from build123d import *

# Parameters (mm, degrees)
F1_DEPTH = 2165
F2_W     = 1270
F2_H     = 45
F3_DEPTH = 40
F4_W     = 925
F4_H     = 2125
F5_DEPTH = 235


with BuildPart() as f1:
    # F0 (on Top) → F1 (new body)
    with BuildSketch(Plane.XY):
        Polygon((0, 255), (0, 0), (1270, 0), (1270, 45), (965, 45), (965, 255), align=None)
    extrude(amount=F1_DEPTH)

    # F2 (on face) → F3 (join)
    with BuildSketch(Plane.XY.offset(2165)):
        with Locations((635, 22.5)):
            Rectangle(F2_W, F2_H)
    extrude(amount=F3_DEPTH)

    # F4 (on face) → F5 (cut)
    with BuildSketch(Plane.XZ):
        with Locations((482.5, 1082.5)):
            Rectangle(F4_W, F4_H)
    extrude(amount=-F5_DEPTH, mode=Mode.SUBTRACT)


solid = f1.part
CAD build for the part. Positions are in the model's coordinates, mm. A direction names the side the tool comes from. Coordinates: 2 decimals unless noted, no trailing zeros. Order: outer loops, then holes, each group sorted by start corner. A loop starts at its lowest first (then second) coordinate and runs counter-clockwise, first axis right, second up.
Item 1: Two-plate mould, pull along Z, no slides. Class faces 1 (the face through (485, 129, 0)), 2 (the face through (1055, 0, 1179)), 3 (the face through (476, 116, 20)), 4 (the face through (476, 151, 2165)): +Z half, -Z half, draft (parallel to the pull), parting line (faces both ways), or undercut.
Check sheet entries:
face 1: -Z half
face 2: draft
face 3: undercut
face 4: +Z half
Item 2: Band-saw the part on B-B on x = 268. List the corners of the cut face in (y, z).
Check sheet entries:
outline: (0, 0) - (255, 0) - (255, 2165) - (45, 2165) - (45, 2205) - (0, 2205) - (0, 2145) - (235, 2145) - (235, 20) - (0, 20) - close
Item 3: Drill centre lines: L1, parallel to Z at x = 707, y = 84; L2, parallel to X at y = 226, z = 1235.5; L3, parallel to Z at x = 943.5, y = 22.5. Where is each one in solid material? Low to high.
Check sheet entries:
L1: z = 0 to 20, 2145 to 2165
L2: x = 0 to 20, 945 to 965
L3: z = 0 to 20, 2145 to 2205
Item 4: Pin check, flat tips, straight feed: pin 1 Ø3 at (y, z) = (84.5, 1675) entering from +X; pin 2 Ø4 at (x, y) = (631.5, 93) entering from +Z. Stop position of each tip, or through.
Check sheet entries:
pin 1: stops at x = 965
pin 2: stops at z = 2165
Item 5: 3-axis set-ups, long thin cutter, end or side, ignore diameter. For faces 5 (the face through (945, 116, 1068)), 6 (the face through (965, 149, 1067)), 7 (the face through (626, 23, 2205)): which of +Z, -Z, +X, -X, +Y, -Y reach the whole face in a straight line?
Check sheet entries:
face 5: -Y
face 6: +Z, -Z, +X, +Y
face 7: +Z, +X, -X, +Y, -Y
Item 6: Band-saw the part on A-A on z = 331. List the corners of the cut face in (x, y), plus the area to 3 significant figures.
Check sheet entries:
outline: (0, 0) - (20, 0) - (20, 235) - (945, 235) - (945, 0) - (1270, 0) - (1270, 45) - (965, 45) - (965, 255) - (0, 255) - close
area: 42,400 mm2
Item 7: Band-saw the part on C-C on y = 139. List the corners of the cut face in (x, z), plus the area to 3 significant figures.
Check sheet entries:
outline: (0, 0) - (965, 0) - (965, 2165) - (0, 2165) - close; hole (20, 20) - (945, 20) - (945, 2145) - (20, 2145) - close
area: 124,000 mm2
